Autodesk Inventor part; units mm, degrees
ref_plane "MSC_PF1" through (0, 0, 0) normal (1, 0, 0) x (0, 1, 0)
ref_plane "MSC_PT1" through (0, 0, 0) normal (0, 0, 1) x (1, 0, 0)
ref_plane "YZ Plane" through (0, 0, 0) normal (1, 0, 0) x (0, 1, 0)
sketch "Sketch7" plane through (0, 0, 0) normal (0, 0, 1) x (1, 0, 0)
  circle A0 centre (0, 0) radius 4.7625 construction
  line L0 (-4.7625, -2.7496) -> (-4.7625, 2.7496)
  line L1 (-4.7625, 2.7496) -> (0, 5.4993)
  line L2 (0, 5.4993) -> (4.7625, 2.7496)
  line L3 (4.7625, 2.7496) -> (4.7625, -2.7496)
  line L4 (4.7625, -2.7496) -> (0, -5.4993)
  line L5 (0, -5.4993) -> (-4.7625, -2.7496)
  dimension "d40" = 9.525
extrude "Extrusion1" add sketch "Sketch7" against normal blind 3.302
sketch "Sketch11" plane through (0, 0, 0) normal (0, 0, 1) x (1, 0, 0)
  line L0 (0, 5.4993) -> (4.7625, 2.7496)
  line L1 (-4.7625, 2.7496) -> (0, 5.4993)
  line L2 (-4.7625, 2.7496) -> (4.7625, -2.7496) construction
  line L3 (-4.7625, -2.7496) -> (4.7625, 2.7496) construction
  point P0 (0, 0)
hole "Hole1" at (0, 0, 0) direction (0, 0, -1) diameter 3.9624 end through all
chamfer "Chamfer1" distance 0.0156 angle 45 2 edges at (0, 1.9812, 0) (0, 1.9812, -3.302)
sketch "Sketch9" plane through (0, 0, 0) normal (1, 0, 0) x (0, 1, 0)
  line L0 (-5.4993, -2.8766) -> (-5.4993, -3.302)
  line L1 (-5.4993, -3.302) -> (-4.7625, -3.302)
  line L2 (-4.7625, -3.302) -> (-5.4993, -2.8766)
  line L3 (0, -3.3871) -> (0, -2.7916)
  line L4 (-5.4993, -3.302) -> (-2.7496, -3.302)
  dimension "d38" = 9.525
  dimension "d41" = 150
revolve "Revolution1" cut sketch "Sketch9" angle 360 about axis through (0, 0, -10) along (0, 0, 1)
sketch "Sketch10" plane through (0, 0, 0) normal (1, 0, 0) x (0, 1, 0)
  line L0 (-5.4993, -0.4254) -> (-5.4993, 0)
  line L1 (-5.4993, 0) -> (-4.7625, 0)
  line L2 (-4.7625, 0) -> (-5.4993, -0.4254)
  line L3 (0, -0.5104) -> (0, 0.0851)
  line L4 (-2.7496, 0) -> (-5.4993, 0)
  dimension "d45" = 9.525
  dimension "d46" = 150
revolve "Revolution2" cut sketch "Sketch10" angle 360 about axis through (0, 0, -10) along (0, 0, 1)
ref_plane "MSC_PF1" through (0, 0, 0) normal (1, 0, 0) x (0, 1, 0)
ref_plane "MSC_PT1" through (0, 0, 0) normal (0, 0, 1) x (1, 0, 0)
equation "\"d38\" = Fbas"
equation "\"d40\" = Fbas"
equation "\"d29\" = Hbas"
equation "\"d63\" = 0.5 * PTC"
equation "\"d45\" = Fbas"
equation "\"Fbas\" = 9.525"
equation "\"Hbas\" = 3.302"
equation "\"NND\" = 4.826"
equation "\"THREADDIA\" = NND"
properties part number "ASME B18.6.3 - 10-32" material "Steel, Mild"
Model file for the job. Use its own axes, mm. Coordinates: 2 decimals unless noted, no trailing zeros. Order: outer loops, then holes, each group sorted by start corner. A loop starts at its lowest first (then second) coordinate and runs counter-clockwise, first axis right, second up. Notation, with made-up numbers: (53, -10) -> (92, -10) arc R18 cw to (92, -4) -> close; hole circle Ø11 at (-5.5, 21). An arc over 180 degrees is marked (long way). Answer as a JSON object with one key per item and string values. Group by question number.
1) Drill centre lines: L1, parallel to X at y = 0, z = -1.1; L2, parallel to Y at x = 1.75, z = -1.9; L3, parallel to Y at x = -0.75, z = -1.15. Where is each one in solid material? Low to high.
2) Flat gauge pin, fed straight in: pin 1 (1.5 mm diameter, centred on x = 3, z = -3, fed in from +Y). Where does the tip first touch, or does it go through?
3) Cut at A-A, the plane z = -2. Write the cut outline in (x, y), then the cut area to 3 significant figures.
Check values:
{
 "1": {"L1": "x = -4.76 to -1.98, 1.98 to 4.76", "L2": "y = -4.49 to -0.93, 0.93 to 4.49", "L3": "y = -5.07 to -1.83, 1.83 to 5.07"},
 "2": {"pin 1": "stops at y = 4.2"},
 "3": {"outline": "(-4.76, -2.75) -> (0, -5.5) -> (4.76, -2.75) -> (4.76, 2.75) -> (0, 5.5) -> (-4.76, 2.75) -> close; hole circle Ø3.96 at (0, 0)", "area": "66.2 mm²"}
}
